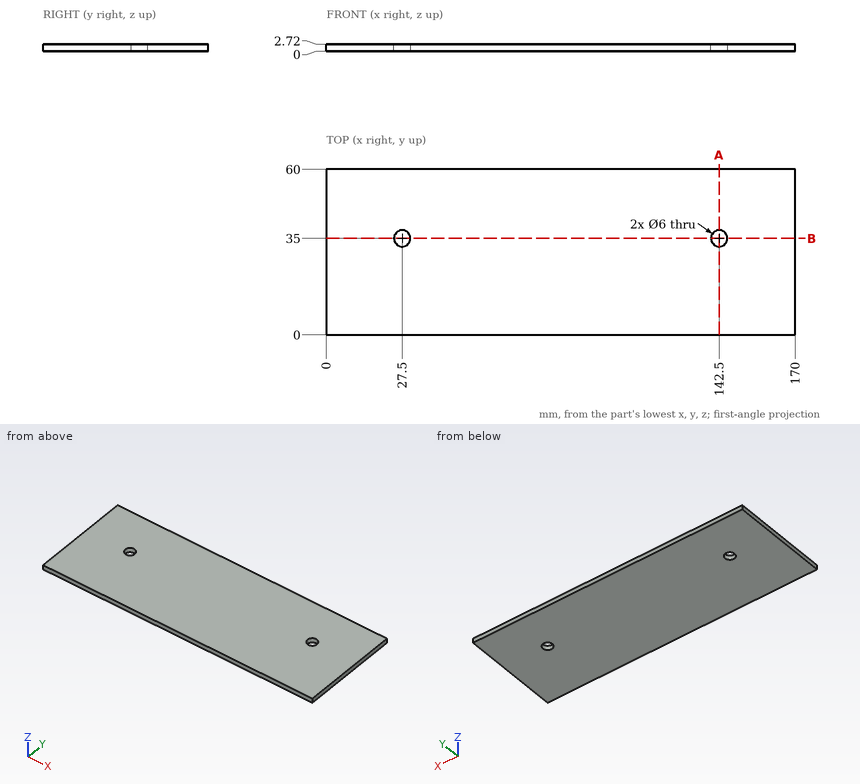
Drawing for the job (mm, zero at the part's lowest x, y, z). Round coordinates to 2 decimals unless told otherwise and drop trailing zeros. Loops run counter-clockwise (first coordinate to the right, second up) from the corner with the lowest first, then second, coordinate; pieces in that order, holes last. Notation, with made-up numbers: M -6,3.25 L 14,3.25 A24 ccw 14,38.25 Z; hole C 25.5,-1.5 d5. An arc over 180 degrees is marked long. Use a Markdown table: item, result. Add a question column.
(1) Drill centre lines: line 1 (Y direction, x = 142.5, z = 1.55); line 2 (X direction, y = 37, z = 1.95). Where is each one in solid material? Low to high.
(2) Cut at B-B (y = 35). Give the cut face in (x, z), and give its area (3 significant figures).
(3) Flat gauge pins, fed straight in: pin 1 (2 mm diameter, centred on x = 51, y = 27.5, fed in from -Z); pin 2 (3.5 mm diameter, centred on x = 142.5, y = 35, fed in from -Z). Where does each tip first touch, or does it go through?
(4) Cut at A-A (x = 142.5). Give the cut face in (y, z), and give its area (3 significant figures).
Geometry says:
| question | item | result |
|---|---|---|
| 1 | line 1 | y = 0 to 32, 38 to 60 |
| 1 | line 2 | x = 0 to 25.26, 29.74 to 140.26, 144.74 to 170 |
| 2 | outline | M 0,0 L 24.5,0 L 24.5,2.72 L 0,2.72 Z; M 30.5,0 L 139.5,0 L 139.5,2.72 L 30.5,2.72 Z; M 145.5,0 L 170,0 L 170,2.72 L 145.5,2.72 Z |
| 2 | area | 430 mm² |
| 3 | pin 1 | stops at z = 0 |
| 3 | pin 2 | passes through |
| 4 | outline | M 0,0 L 32,0 L 32,2.72 L 0,2.72 Z; M 38,0 L 60,0 L 60,2.72 L 38,2.72 Z |
| 4 | area | 147 mm² |
